Verification items for this drawing (mm, ordinates from the low corner). Coordinates: 2 decimals unless noted, no trailing zeros. Order: outer loops, then holes, each group sorted by start corner. A loop starts at its lowest first (then second) coordinate and runs counter-clockwise, first axis right, second up. Notation, with made-up numbers: M 89,-18.75 L 147,-18.75 A18 cw 147,-8.75 Z; hole C 60.5,14 d11. An arc over 180 degrees is marked long. Return JSON: item names as keys, results as strings. Group by question number.
1. Section check C-C, the plane x = 17.75. Record the cut outline in (y, z), plus the area to 3 significant figures.
2. Section check A-A, the plane x = 20.75. Record the cut outline in (y, z).
3. Gauge pin test, flat ends, axial feed: pin 1 (1.5 mm diameter, centred on y = 4, z = 11, fed in from -X); pin 2 (1 mm diameter, centred on x = 5, y = 2, fed in from +Z) (1 decimal); pin 3 (1 mm diameter, centred on x = 14, y = 2, fed in from -Z). Record the tip position at first contact, or that the pin passes through.
4. Mould release check, pull along Z, two halves, no side actions. Record for the marked faces 1, 2, 3 and 4: +Z half, -Z half, draft (parallel to the pull), parting line (faces both ways), or undercut.
5. Material ranges on line 1 along X through (y, z) = (3.25, 24.5); line 2 along Z through (x, y) = (12.5, 3.85) (1 decimal); line 3 along Z through (x, y) = (24, 0.75) (1 decimal), recorded low to high.
6. Section check D-D, the plane z = 43.5. Record the cut outline in (x, y), plus the area to 3 significant figures.
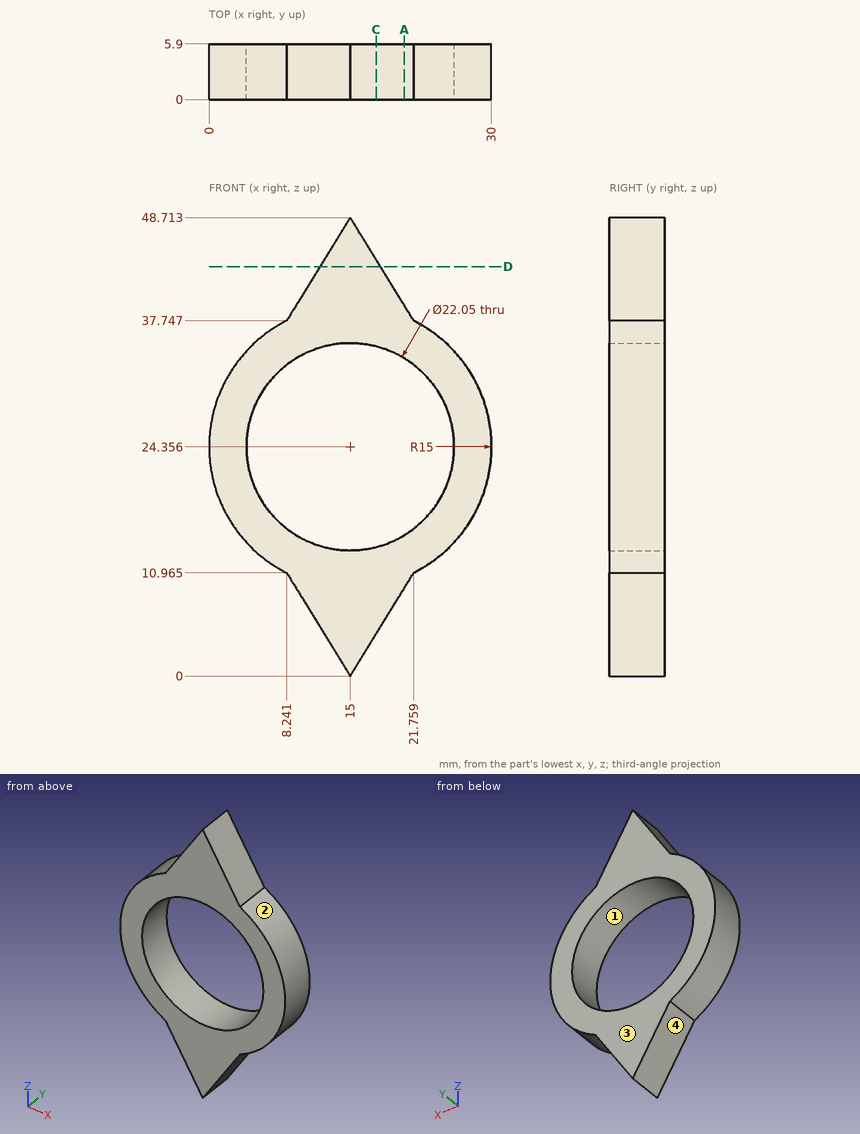
Answers follow:
{
 "1": {"outline": "M 0,4.46 L 5.9,4.46 L 5.9,13.68 L 0,13.68 Z; M 0,35.03 L 5.9,35.03 L 5.9,44.25 L 0,44.25 Z", "area": "109 mm^2"},
 "2": {"outline": "M 0,9.33 L 5.9,9.33 L 5.9,14.95 L 0,14.95 Z; M 0,33.76 L 5.9,33.76 L 5.9,39.38 L 0,39.38 Z"},
 "3": {"pin 1": "x = 6.87", "pin 2": "z = 36", "pin 3": "z = 0.81"},
 "4": {"face 1": "undercut", "face 2": "parting line", "face 3": "draft", "face 4": "-Z half"},
 "5": {"line 1": "0 to 3.98, 26.02 to 30", "line 2": "4.1 to 13.6, 35.1 to 44.7", "line 3": "12.4 to 18, 30.7 to 36.4"},
 "6": {"outline": "M 11.79,0 L 18.21,0 L 18.21,5.9 L 11.79,5.9 Z", "area": "37.9 mm^2"}
}
